from build123d import *

# Parameters (mm, degrees)
BOSS_EXTRUDE1_DEPTH  = 1.016
CUT_EXTRUDE1_DEPTH   = 1.016
CIRPATTERN1_COUNT    = 6
SKETCH3_W            = 3
SKETCH3_H            = 3
BOSS_EXTRUDE2_DEPTH  = 3
FILLET1_R            = 0.0508
FILLET2_R            = 0.0508
FILLET3_R            = 0.0508
FILLET4_R            = 0.0508
BOSS_EXTRUDE3_DEPTH  = 6.35
CIRPATTERN2_COUNT    = 2
CIRPATTERN2_ANGLE    = 60
BOSS_EXTRUDE4_DEPTH  = 1.016
BOSS_EXTRUDE5_DEPTH  = 1.016
MIRROR1_COPY_1_DEPTH = 6.35


with BuildPart() as part:
    # Sketch1 → Boss-Extrude1 (new body)
    with BuildSketch(Plane(origin=(0, 0, 0), x_dir=(1, 0, 0), z_dir=(0, 1, 0))):
        Polygon((5.741228812, 9.9441), (-5.741228812, 9.9441), (-11.482457624, 0), (-5.741228812, -9.9441), (5.741228812, -9.9441), (11.482457624, 0), align=None)
    extrude(amount=BOSS_EXTRUDE1_DEPTH)

    # Sketch2 → Cut-Extrude1 (cut)
    with BuildSketch(Plane(origin=(0, 1.016, 0), x_dir=(1, 0, 0), z_dir=(0, 1, 0))):
        with BuildLine():
            Line((9.525, 1.5875), (13.137780832, 1.5875))
            Line((13.137780832, 1.5875), (13.137780832, -1.5875))
            Line((13.137780832, -1.5875), (9.525, -1.5875))
            ThreePointArc((9.525, -1.5875), (7.9375, 0), (9.525, 1.5875))
        make_face()
    cut_extrude1 = extrude(amount=-CUT_EXTRUDE1_DEPTH, mode=Mode.SUBTRACT)

    # CirPattern1: Cut-Extrude1 ×6 about axis
    cirpattern1_axis = Axis((0, 0, 0), (0, 1, 0))
    for i in range(1, CIRPATTERN1_COUNT):
        add(cut_extrude1.rotate(cirpattern1_axis, i * 360 / CIRPATTERN1_COUNT), mode=Mode.SUBTRACT)

    # Sketch3 → Boss-Extrude2 (add)
    with BuildSketch(Plane(origin=(0, 1.016, 0), x_dir=(1, 0, 0), z_dir=(0, 1, 0))):
        Rectangle(SKETCH3_W, SKETCH3_H)
    extrude(amount=BOSS_EXTRUDE2_DEPTH)

    # Fillet1
    fillet1_edges = [part.edges().sort_by_distance(p)[0] for p in [
        (1.5, 2.516, 1.5),
    ]]
    fillet(fillet1_edges, radius=FILLET1_R)

    # Fillet2
    fillet2_edges = [part.edges().sort_by_distance(p)[0] for p in [
        (-1.5, 2.516, -1.5),
    ]]
    fillet(fillet2_edges, radius=FILLET2_R)

    # Fillet3
    fillet3_edges = [part.edges().sort_by_distance(p)[0] for p in [
        (1.5, 2.516, -1.5),
    ]]
    fillet(fillet3_edges, radius=FILLET3_R)

    # Fillet4
    fillet4_edges = [part.edges().sort_by_distance(p)[0] for p in [
        (-1.5, 2.516, 1.5),
    ]]
    fillet(fillet4_edges, radius=FILLET4_R)

    # Sketch5 → Boss-Extrude3 (add)
    with BuildSketch(Plane(origin=(-5.734684765, 0, 3.310921793), x_dir=(0.5, 0, 0.866025404), z_dir=(-0.866025404, 0, 0.5))):
        with BuildLine():
            ThreePointArc((-1.520793442, 1.016), (0.422306558, 2.9591), (2.365406558, 1.016))
            Line((2.365406558, 1.016), (-1.520793442, 1.016))
        make_face()
    boss_extrude3 = extrude(amount=BOSS_EXTRUDE3_DEPTH)

    # CirPattern2: Boss-Extrude3 ×2 about axis
    cirpattern2_axis = Axis((0, 4.2168, 0), (0, -1, 0))
    for i in range(1, CIRPATTERN2_COUNT):
        add(boss_extrude3.rotate(cirpattern2_axis, i * CIRPATTERN2_ANGLE / (CIRPATTERN2_COUNT - 1)))

    # Sketch7 → Boss-Extrude4 (add)
    with BuildSketch(Plane.XZ.offset(-1.016)):
        Polygon((-11.9943428, 5.168876038), (-9.372239939, 3.655004245), (-7.429139939, 7.020552169), (-10.0512428, 8.534423962), align=None)
    boss_extrude4 = extrude(amount=BOSS_EXTRUDE4_DEPTH)

    # Sketch8 → Boss-Extrude5 (add)
    with BuildSketch(Plane.XZ.offset(-1.016)):
        Polygon((-10.473549358, -7.802967548), (-7.851446497, -6.289095755), (-9.794546497, -2.923547831), (-12.416649358, -4.437419623), align=None)
    boss_extrude5 = extrude(amount=BOSS_EXTRUDE5_DEPTH)

    # Mirror1: Boss-Extrude5, Boss-Extrude4, Boss-Extrude3 across plane
    add(boss_extrude5.mirror(Plane(origin=(0, 0, 0), x_dir=(0, 0, 1), z_dir=(1, 0, 0))))
    add(boss_extrude4.mirror(Plane(origin=(0, 0, 0), x_dir=(0, 0, 1), z_dir=(1, 0, 0))))
    add(boss_extrude3.mirror(Plane(origin=(0, 0, 0), x_dir=(0, 0, 1), z_dir=(1, 0, 0))))

    # Mirror1 copy 1 sketch → Mirror1 copy 1 (add)
    with BuildSketch(Plane(origin=(5.734684765, 0, -3.310921793), x_dir=(0.5, 0, 0.866025404), z_dir=(0.866025404, 0, -0.5))):
        with BuildLine():
            ThreePointArc((-1.520793442, -1.016), (0.422306558, -2.9591), (2.365406558, -1.016))
            Line((2.365406558, -1.016), (-1.520793442, -1.016))
        make_face()
    extrude(amount=MIRROR1_COPY_1_DEPTH)


solid = part.part
CAD build for the part. Positions are in the model's coordinates, mm. A direction names the side the tool comes from. Coordinates: 2 decimals unless noted, no trailing zeros. Loops run counter-clockwise (first coordinate to the right, second up) from the corner with the lowest first, then second, coordinate; pieces in that order, holes last. Notation, with made-up numbers: (35, 58.5) - (46, 58.5) arc R12 cw to (46, 63.5) - close; hole circle Ø4 at (22, 30). An arc over 180 degrees is marked (long way). Use one line per item in the form item = value. Start each with the question number.
1) Tool access for faces 4 (the face through (-10.175, 0.501, -2.265)), 5 (the face through (3.644, 0.515, -9.487)), 6 (the face through (0, 2, -1.5)): list every direction of +Z, -Z, +X, -X, +Y, -Y with a clear straight run to the whole face (end or side of a thin tool).
2) Two-plate mould, pull along Z, no slides. Class faces 1 (the face through (10.186, 0.501, -2.246)), 2 (the face through (-0.1, 0.5, 9.944)), 3 (the face through (-9.181, 0.515, -7.057)): +Z half, -Z half, draft (parallel to the pull), parting line (faces both ways), or undercut.
3) Flat gauge pins, fed straight in: pin 1 (1.4 mm diameter, centred on y = 2, z = 0.5, fed in from -X); pin 2 (2 mm diameter, centred on x = 1.5, z = 7.5, fed in from +Y); pin 3 (2 mm diameter, centred on y = 0.5, z = -1.5, fed in from +X). Where does each tip first touch, or does it go through?
4) Band-saw the part on B-B (y = 2.35). Give the cut face in (x, z).
5) Band-saw the part on A-A (x = 0.5). Give the cut face in (y, z).
6) Band-saw the part on C-C (z = 0). Give the cut face in (x, y).
7) Drill centre lines: L1, parallel to Z at x = -9.5, y = 0.3; L2, parallel to Y at x = 6, z = -1.5; L3, parallel to X at y = 1.3, z = -3. Where is each one in solid material? Low to high. Write a range as from..to.
Check values:
q1.face_4 = -X, +Y, -Y
q1.face_5 = +X, +Y, -Y
q1.face_6 = -Z, +Y
q2.face_1 = undercut
q2.face_2 = +Z half
q2.face_3 = -Z half
q3.pin_1 = -1.5
q3.pin_2 = 1.02
q3.pin_3 = 10.57
q4.outline = (-12.15, -4.9) - (-10.74, -7.34) - (-5.24, -4.17) - (-6.65, -1.72) - close; (-11.73, 5.63) - (-6.23, 2.45) - (-4.82, 4.9) - (-10.32, 8.08) - close; (-1.5, -1.45) arc R0.05 ccw to (-1.45, -1.5) - (1.45, -1.5) arc R0.05 ccw to (1.5, -1.45) - (1.5, 1.45) arc R0.05 ccw to (1.45, 1.5) - (-1.45, 1.5) arc R0.05 ccw to (-1.5, 1.45) - close; (4.82, 4.9) - (6.23, 2.45) - (11.73, 5.63) - (10.32, 8.08) - close; (5.24, -4.17) - (10.74, -7.34) - (12.15, -4.9) - (6.65, -1.72) - close
q5.outline = (0, -9.94) - (1.02, -9.94) - (1.02, -1.5) - (4.02, -1.5) - (4.02, 1.5) - (1.02, 1.5) - (1.02, 9.94) - (0, 9.94) - close
q6.outline = (-7.94, 0) - (7.94, 0) - (7.94, 1.02) - (1.5, 1.02) - (1.5, 4.02) - (-1.5, 4.02) - (-1.5, 1.02) - (-7.94, 1.02) - close
q7.L1 = -7.24..-1.59, 1.59..3.43, 3.73..8.22
q7.L2 = 0..1.02
q7.L3 = -9.89..-5.91, 5.91..9.89
